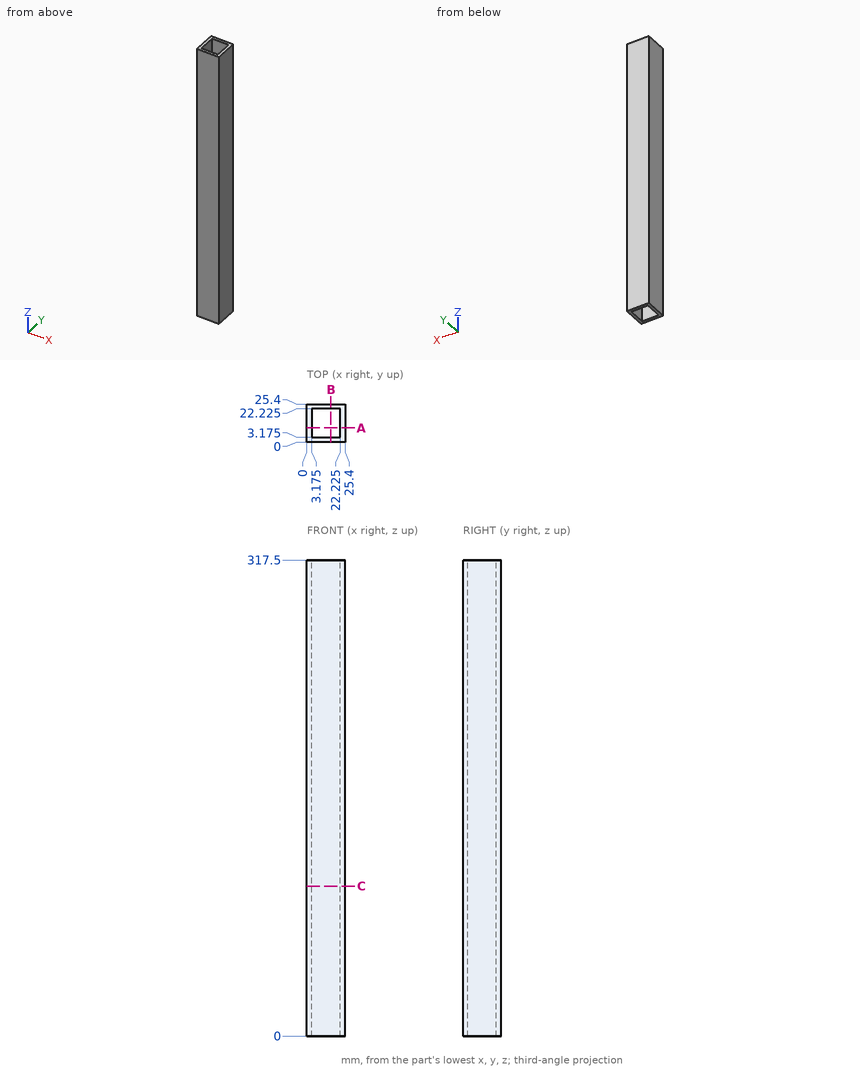
Answer from the drawing. Dimensions are ordinates in mm from the lowest x, y and z of the part. Round coordinates to 2 decimals unless told otherwise and drop trailing zeros. Order: outer loops, then holes, each group sorted by start corner. A loop starts at its lowest first (then second) coordinate and runs counter-clockwise, first axis right, second up. Notation, with made-up numbers: (53.25, -17.5) - (58.25, -17.5) arc R13 cw to (58.25, -11.5) - close; hole circle Ø9 at (79, 58.5). An arc over 180 degrees is marked (long way). Put each result on its own line as item: value. Start each with the question number.
(1) Given P1, Ø15, axis at x = 14.5, z = 179, coming from the -Y side, flat-ended and moving along its own axis, determine where the tip first touches the part or whether it passes through.
(2) A straight line is drawn through the part: probe 1 along Y at (x, z) = (21, 110.5) (3 decimals). Find the intervals that lie inside material, in ascending order. Write a range as from..to.
(3) Find section A-A (y = 9.5). Give the vertices of the cut face in (x, z) (3 decimals).
(4) Find section C-C (z = 100). Give the vertices of the cut face in (x, y) (3 decimals).
Reply:
1. P1: y = 0
2. probe 1: 0..3.175, 22.225..25.4
3. outline: (0, 0) - (3.175, 0) - (3.175, 317.5) - (0, 317.5) - close; (22.225, 0) - (25.4, 0) - (25.4, 317.5) - (22.225, 317.5) - close
4. outline: (0, 0) - (25.4, 0) - (25.4, 25.4) - (0, 25.4) - close; hole (3.175, 3.175) - (22.225, 3.175) - (22.225, 22.225) - (3.175, 22.225) - close
